Study the drawing (mm; zero at the part's minimum x, y, z) and answer. Coordinates: 2 decimals unless noted, no trailing zeros. Order: outer loops, then holes, each group sorted by start corner. A loop starts at its lowest first (then second) coordinate and runs counter-clockwise, first axis right, second up. Notation, with made-up numbers: M -6.5,82 L 47.5,82 A25 cw 47.5,110 Z; hole C 14,-21 d9. An arc over 180 degrees is marked long. Use a Markdown table: item, result. Add a question column.
1) Find section A-A on x = 427.5. Write down the section's boundary in (y, z).
2) Each of these flat-tipped pins is pushed along its axis until it touches: pin 1 Ø6.5 at (y, z) = (296.5, 6.5) entering from +X; pin 2 Ø6 at (x, z) = (86, 11) entering from +Y. Where does it stop, or does it pass through?
3) Find the intervals of material crossed by probe 1 along X at (y, z) = (295.5, 9); probe 2 along Y at (x, z) = (317.5, 1.5); probe 3 along Y at (x, z) = (27.5, 11), in increasing order. Write a range as [from, to].
4) Find section B-B on y = 510. Write down the section's boundary in (x, z), plus the area to 3 significant figures.
5) Find section C-C on z = 9. Write down the section's boundary in (x, y), plus the area to 3 significant figures.
6) Find section D-D on x = 126.5. Write down the section's boundary in (y, z), plus the area to 3 significant figures.
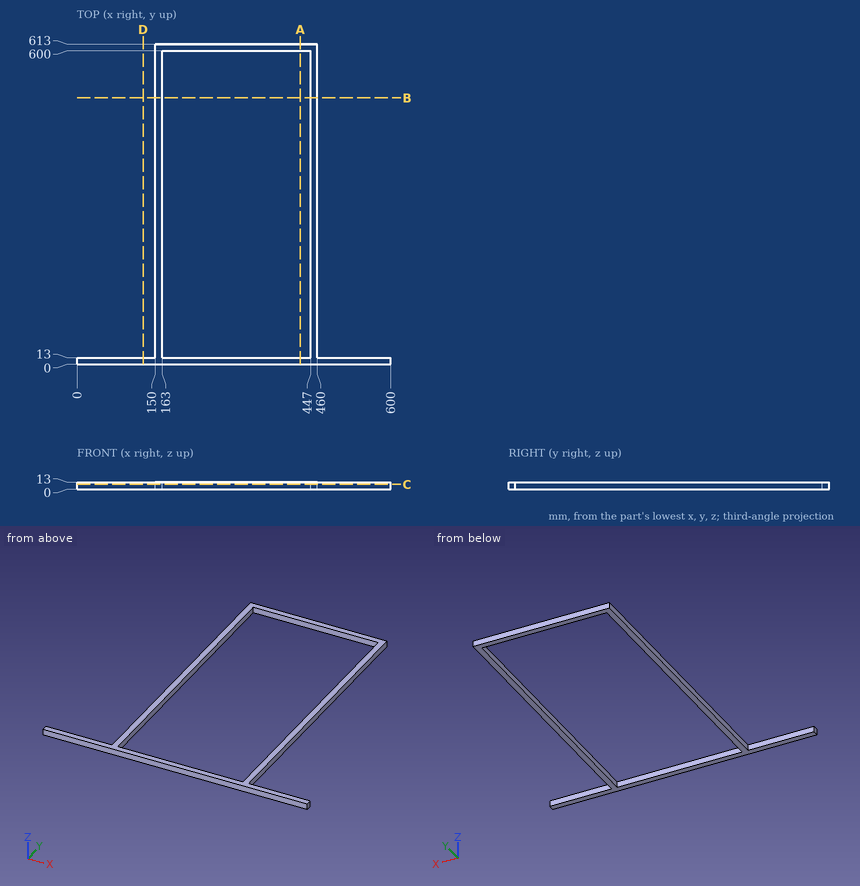
Check result:
| question | item | result |
|---|---|---|
| 1 | outline | M 0,0 L 13,0 L 13,13 L 0,13 Z; M 600,0 L 613,0 L 613,13 L 600,13 Z |
| 2 | pin 1 | stops at x = 460 |
| 2 | pin 2 | stops at y = 13 |
| 3 | probe 1 | x = [150, 163], [447, 460] |
| 3 | probe 2 | y = [0, 13], [600, 613] |
| 3 | probe 3 | y = [0, 13] |
| 4 | outline | M 150,0 L 163,0 L 163,13 L 150,13 Z; M 447,0 L 460,0 L 460,13 L 447,13 Z |
| 4 | area | 338 mm2 |
| 5 | outline | M 0,0 L 600,0 L 600,13 L 460,13 L 460,613 L 150,613 L 150,13 L 0,13 Z; hole M 163,13 L 447,13 L 447,600 L 163,600 Z |
| 5 | area | 27,100 mm2 |
| 6 | outline | M 0,0 L 13,0 L 13,13 L 0,13 Z |
| 6 | area | 169 mm2 |
